Geometry: final body of the model. Coordinates: model frame, mm. A direction names the side the tool comes from. Coordinates: 2 decimals unless noted, no trailing zeros. Order: outer loops, then holes, each group sorted by start corner. A loop starts at its lowest first (then second) coordinate and runs counter-clockwise, first axis right, second up. Notation, with made-up numbers: (-8, -14.75) -> (38, -14.75) arc R20 ccw to (38, 3.25) -> close; hole circle Ø3 at (85.25, 26). An arc over 180 degrees is marked (long way). Answer in a Markdown table with one row per item. Add a question column.
1) Set-up query: faces 1 (the face through (-13, 3.175, 22)), 2 (the face through (0, 2, 35)). Return all of +Z, -Z, +X, -X, +Y, -Y with unobstructed straight access to the full face (end or side cutting, diameter ignored); none if empty.
2) Ray query, line 1 (Y direction, x = -1.5, z = 35) (3 decimals); line 2 (Z direction, x = -19.75, y = 15.25) (3 decimals); line 3 (Z direction, x = -5.25, y = 4.75). Return the intervals inside material, ascending. Write a range as from..to.
3) Section query C-C on y = 19.5. Return the cut outline in (x, z) (3 decimals).
4) Section query A-A on x = -22.5. Return the cut outline in (y, z) (1 decimal), then the cut area to 3 significant figures.
5) Contact query for a flat-ended pin moving along its axis: P1, Ø1, axis at x = -20.5, z = 29, coming from the -Y side. Output: stop coordinate, or through.
6) Section query B-B on z = 22.5. Return the cut outline in (x, y) (3 decimals), then the cut area to 3 significant figures.
Autodesk Inventor part; units mm, degrees
ref_plane "YZ Plane" through (0, 0, 0) normal (1, 0, 0) x (0, 1, 0)
ref_plane "XZ Plane" through (0, 0, 0) normal (0, 1, 0) x (-1, 0, 0)
ref_plane "XY Plane" through (0, 0, 0) normal (0, 0, 1) x (1, 0, 0)
sketch "Sketch1" plane through (0, 0, 0) normal (0, 1, 0) x (-1, 0, 0)
  line L0 (0, 0) -> (25.4, 0)
  line L1 (25.4, 0) -> (25.4, 50.8)
  line L2 (25.4, 50.8) -> (0, 50.8)
  line L3 (0, 50.8) -> (0, 0)
  dimension "d0" = 25.4
  dimension "d1" = 50.8
extrude "Plate1" add sketch "Sketch1" along normal blind 3.175
sketch "Sketch2" plane through (0, 0, 47.625) normal (0, 0, 1) x (1, 0, 0)
  line L0 (-25.4, 0) -> (0, 0)
  line L1 (0, 0) -> (0, 25.4)
  line L2 (0, 25.4) -> (-25.4, 25.4)
  line L3 (-25.4, 25.4) -> (-25.4, 0)
edge flange "Flange1" height 25.4 angle 90 thickness 3.175 bend radius 4.7625 thickness toward (0, 0, 1) relief tear relief width 3.175 relief depth 1.5875 edges at (-12.7, 3.175, 50.8) wall of the first edge with corners at (-25.4, 0, 47.625) (0, 0, 47.625) (0, 25.4, 47.625) (-25.4, 25.4, 47.625)
bend "Bend1"
corner "Corner1"
equation "\"d2\" = Thickness"
equation "\"d3\" = BendReliefWidth"
equation "\"d4\" = BendReliefDepth"
equation "\"d5\" = MinimumRemnant"
equation "\"d6\" = TransitionRadius"
equation "\"d9\" = BendRadius"
equation "\"d10\" = CornerReliefSize"
equation "\"d11\" = GapSize"
equation "\"d12\" = JacobiRadiusSize"
equation "\"BendRadius\" = 1.5 * Thickness"
equation "\"BendReliefWidth\" = Thickness"
equation "\"BendReliefDepth\" = 0.5 * Thickness"
equation "\"CornerReliefSize\" = 4 * Thickness"
equation "\"MinimumRemnant\" = 2 * Thickness"
equation "\"TransitionRadius\" = BendRadius"
equation "\"JacobiRadiusSize\" = BendRadius"
equation "\"GapSize\" = Thickness"
properties part number "200557" material "Aluminum 5052 H32"
Result:
| question | item | result |
|---|---|---|
| 1 | face 1 | -Z, +X, -X, +Y |
| 1 | face 2 | +Z, -Z, +X, +Y, -Y |
| 2 | line 1 | 0..3.175 |
| 2 | line 2 | 47.625..50.8 |
| 2 | line 3 | 46.4..50.13 |
| 3 | outline | (-25.4, 47.625) -> (0, 47.625) -> (0, 50.8) -> (-25.4, 50.8) -> close |
| 4 | outline | (0, 0) -> (3.2, 0) -> (3.2, 42.9) arc R4.8 cw to (7.9, 47.6) -> (25.4, 47.6) -> (25.4, 50.8) -> (7.9, 50.8) arc R7.9 ccw to (0, 42.9) -> close |
| 4 | area | 223 mm2 |
| 5 | P1 | y = 0 |
| 6 | outline | (-25.4, 0) -> (0, 0) -> (0, 3.175) -> (-25.4, 3.175) -> close |
| 6 | area | 80.6 mm2 |
